```python
from build123d import *

# Parameters (mm, degrees)
F0_W        = 14
F0_H        = 30
F0_R        = 1
F1_DEPTH    = 4
F3_DEPTH    = 8
F4_DEPTH    = 4.001
F5_R        = 1
F6_T1_DEPTH = 12


# Not quite as in the source:
# - a fillet or chamfer that OpenCascade refuses, or shapes differently, is made with other operations: its cross-section is extruded or revolved along the edge and cut away or added


with BuildPart() as f1:
    # F0 (on Top) → F1 (new body)
    with BuildSketch(Plane.XY):
        with Locations((0, 15)):
            Rectangle(F0_W, F0_H)
        with Locations((0, 3)):
            Circle(F0_R, mode=Mode.SUBTRACT)
    extrude(amount=F1_DEPTH)

    # F2 (on face) → F3 (join)
    with BuildSketch(Plane.XY.offset(4)):
        Polygon((-5, 27), (-5, 30), (-7, 30), (-7, 26), (7, 26), (7, 30), (5, 30), (5, 27), align=None)
    extrude(amount=F3_DEPTH)

    # F4 (cut, through all): a face of the model
    f4_faces = [f1.faces().sort_by_distance(p)[0] for p in [
        (0, 28.5, 4),
    ]]
    extrude(f4_faces, amount=-F4_DEPTH, mode=Mode.SUBTRACT)

    # F5
    f5_edges = [f1.edges().sort_by_distance(p)[0] for p in [
        (-7, 30, 6),
        (7, 30, 6),
        (-7, 28, 12),
        (7, 28, 12),
        (7, 15, 0),
        (-7, 15, 0),
        (-7, 13, 4),
        (7, 13, 4),
    ]]
    fillet(f5_edges, radius=F5_R)

    # F6: fillet of radius 2 on 2 edges, made by hand

    # F6_s2 → F6_t1 (cut)
    with BuildSketch(Plane.XY.offset(-4)):
        with BuildLine():
            ThreePointArc((-7, 2), (-6.4142135624, 0.5857864376), (-5, 0))
            Line((-5, 0), (-7, 0))
            Line((-7, 0), (-7, 2))
        make_face()
        with BuildLine():
            ThreePointArc((5, 0), (6.4142135624, 0.5857864376), (7, 2))
            Line((7, 2), (7, 0))
            Line((7, 0), (5, 0))
        make_face()
    extrude(amount=F6_T1_DEPTH, mode=Mode.SUBTRACT)


solid = f1.part
```
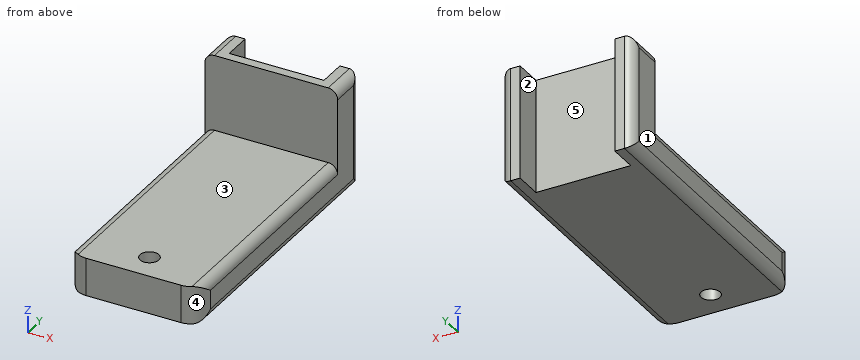
The model under review builds one solid part; all positions refer to its coordinate system, in mm. Face numbers are marked on the shaded views. A direction names the side the tool comes from. Give positions to 0.01 mm unless a question says otherwise; leave off trailing zeros. Write each loop counter-clockwise with the first axis right and the second up, starting at its lowest first coordinate (ties: lowest second). Pieces come first, ordered by that corner, then holes.
(1) Consider section C-C, the plane y = 20.5. Give the boundary of the cut face in (x, z).
(2) Consider section D-D, the plane x = -3.25. Give the boundary of the cut face in (y, z), and give its area (3 significant figures).
(3) Consider section A-A, the plane z = 2.5. Give the boundary of the cut face in (x, y).
(4) Tool access review of the marked faces 1 and 2: name each direction out of +Z, -Z, +X, -X, +Y, -Y from which nothing blocks a thin tool from reaching the whole face with its end or side.
(5) For P1, Ø1, axis at x = 3.5, z = 7, coming from the +Y side; P2, Ø3.5, axis at x = -2, y = 17.5, coming from the +Z side; P3, Ø2.5, axis at x = 0, z = 8, coming from the -Y side, all flat-tipped, find the tip position at first contact; note any pin that passes through.
(6) To check wall thickness, follow L1, parallel to Y at x = 0, z = 1.75; L2, parallel to Z at x = 3.75, y = 6.5; L3, parallel to Y at x = 4, z = 2.5. State the ranges of each line that lie inside material, in increasing order.
(7) Consider section B-B, the plane y = 3. Give the boundary of the cut face in (x, z), and give its area (3 significant figures).
(8) The part is to be moulded in two halves that separate along X. For the marked faces 3, 4 and 5, say which applies: released by +X, released by -X, zero draft, split by the parting line, or undercut.
Returned:
1. outline: (-7, 1) arc R1 ccw to (-6, 0) - (6, 0) arc R1 ccw to (7, 1) - (7, 3) arc R1 ccw to (6, 4) - (-6, 4) arc R1 ccw to (-7, 3) - close
2. outline: (0, 0) - (27, 0) - (27, 12) - (26, 12) - (26, 4) - (0, 4) - close
2. area: 116 mm2
3. outline: (-7, 2) arc R2 ccw to (-5, 0) - (5, 0) arc R2 ccw to (7, 2) - (7, 29) arc R1 ccw to (6, 30) - (5, 30) - (5, 27) - (-5, 27) - (-5, 30) - (-6, 30) arc R1 ccw to (-7, 29) - close; hole circle Ø2 at (0, 3)
4. face 1: +Z, -Z, -X, +Y, -Y
4. face 2: +Z, -Z, +Y
5. P1: stops at y = 27
5. P2: stops at z = 4
5. P3: stops at y = 26
6. L1: y = 0 to 2, 4 to 27
6. L2: z = 0 to 4
6. L3: y = 0 to 27
7. outline: (-7, 1) arc R1 ccw to (-6, 0) - (-1, 0) - (-1, 4) - (-6, 4) arc R1 ccw to (-7, 3) - close; (1, 0) - (6, 0) arc R1 ccw to (7, 1) - (7, 3) arc R1 ccw to (6, 4) - (1, 4) - close
7. area: 47.1 mm2
8. face 3: zero draft
8. face 4: released by +X
8. face 5: undercut
